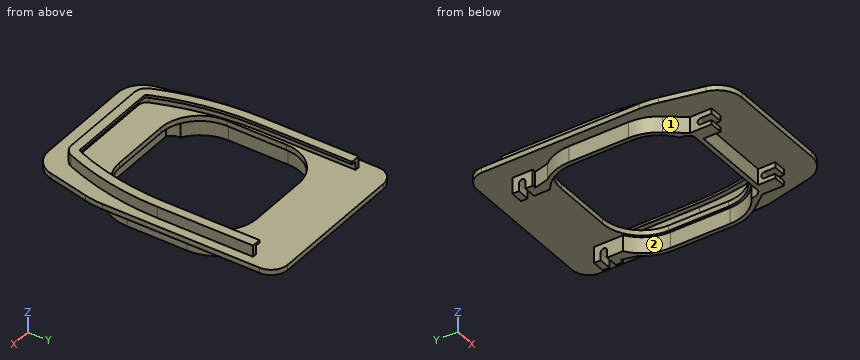
Autodesk Inventor part; units mm, degrees
ref_plane "YZ Plane" through (0, 0, 0) normal (1, 0, 0) x (0, 1, 0)
ref_plane "XZ Plane" through (0, 0, 0) normal (0, 1, 0) x (-1, 0, 0)
ref_plane "XY Plane" through (0, 0, 0) normal (0, 0, 1) x (1, 0, 0)
sketch "Skizze1" plane through (0, 0, 0) normal (0, 0, 1) x (1, 0, 0)
  line L0 (-33.4, 0) -> (33.4, 0)
  line L1 (41.4, -8) -> (41.4, -84.0456)
  line L2 (40.4201, -92.8453) -> (35.956, -112.6399)
  line L3 (24.25, -122) -> (-24.25, -122)
  line L4 (-35.956, -112.6399) -> (-40.4201, -92.8453)
  line L5 (-41.4, -84.0456) -> (-41.4, -8)
  line L6 (0, 0) -> (0, -122) construction
  arc A0 (-41.4, -84.0456) -> (-40.4201, -92.8453) centre (-1.4, -84.0456) ccw
  arc A1 (40.4201, -92.8453) -> (41.4, -84.0456) centre (1.4, -84.0456) ccw
  arc A2 (-35.956, -112.6399) -> (-24.25, -122) centre (-24.25, -110) ccw
  arc A3 (24.25, -122) -> (35.956, -112.6399) centre (24.25, -110) ccw
  arc A4 (-33.4, 0) -> (-41.4, -8) centre (-33.4, -8) ccw
  arc A5 (41.4, -8) -> (33.4, 0) centre (33.4, -8) ccw
  point P0 (33.8452, -122)
  point P1 (-33.8452, -122)
  point P2 (-41.4, -88.5)
  dimension "d1" = 82.8
  dimension "d2" = 122
  dimension "d3" = 33.5
  dimension "d4" = 40
  dimension "d5" = 12
  dimension "d6" = 8
  dimension "d15" = 48.5
extrude "Extrusion1" add sketch "Skizze1" along normal blind 2.6
sketch "Skizze2" plane through (0, 0, 2.6) normal (0, 0, 1) x (1, 0, 0)
  line L0 (-36.8, -14.4) -> (-36.8, -60.5202)
  arc A0 (-36.8, -60.5202) -> (-27.5742, -108.62) centre (93.2, -60.5202) ccw
  line L1 (-22, -112.4) -> (22, -112.4)
  line L2 (36.8, -14.4) -> (36.8, -60.5202)
  arc A1 (27.5742, -108.62) -> (36.8, -60.5202) centre (-93.2, -60.5202) ccw
  line L3 (-36.8, -60.5202) -> (36.8, -60.5202) construction
  line L4 (-36.8, -14.4) -> (36.8, -14.4) construction
  line L5 (0, 0) -> (0, -122) construction
  line L6 (-24.25, -122) -> (24.25, -122) construction
  arc A2 (-27.5742, -108.62) -> (-22, -112.4) centre (-22, -106.4) ccw
  arc A3 (22, -112.4) -> (27.5742, -108.62) centre (22, -106.4) ccw
  line L7 (41.4, -84.0456) -> (41.4, -8) construction
  line L8 (-41.4, -8) -> (-41.4, -84.0456) construction
  line L9 (-34.8, -60.5202) -> (-34.8, -14.4)
  line L10 (34.8, -14.4) -> (34.8, -60.5202)
  arc A4 (25.7161, -107.88) -> (34.8, -60.5202) centre (-93.2, -60.5202) ccw
  arc A5 (22, -110.4) -> (25.7161, -107.88) centre (22, -106.4) ccw
  line L11 (22, -110.4) -> (-22, -110.4)
  arc A6 (-25.7161, -107.88) -> (-22, -110.4) centre (-22, -106.4) ccw
  arc A7 (-34.8, -60.5202) -> (-25.7161, -107.88) centre (93.2, -60.5202) ccw
  line L12 (-36.8, -14.4) -> (-34.8, -14.4)
  line L13 (34.8, -14.4) -> (36.8, -14.4)
  point P0 (-25.9993, -112.4)
  point P1 (25.9993, -112.4)
  point P2 (0, -14.4)
  dimension "d9" = 6
  dimension "d10" = 6
  dimension "d11" = 130
  dimension "d12" = 4.6
  dimension "d13" = 9.6
  dimension "d14" = 44
  dimension "d16" = 14.4
  dimension "d17" = 2
extrude "Extrusion2" add sketch "Skizze2" along normal blind 5.5
sketch "Skizze3" plane through (-36.8, -14.4, 2.6) normal (0, 1, 0) x (1, 0, 0)
  line L0 (2, -4.2) -> (4.5, -4.2)
  line L1 (4.5, -4.2) -> (4.5, -5.5)
  line L2 (4.5, -5.5) -> (2, -5.5)
  line L3 (2, -5.5) -> (2, -4.2)
  line L4 (0, 0) -> (0, -5.5)
  point P0 (36.8, 2.6)
  dimension "d20" = 4.5
  dimension "d21" = 1.3
sketch "Skizze4" plane through (0, 0, 8.1) normal (0, 0, 1) x (1, 0, 0)
  line L0 (-34.8, -60.5202) -> (-34.8, -14.4)
  arc A0 (-34.8, -60.5202) -> (-25.7161, -107.88) centre (93.2, -60.5202) ccw
  arc A1 (-25.7161, -107.88) -> (-22, -110.4) centre (-22, -106.4) ccw
  line L1 (22, -110.4) -> (-22, -110.4)
  arc A2 (22, -110.4) -> (25.7161, -107.88) centre (22, -106.4) ccw
  arc A3 (25.7161, -107.88) -> (34.8, -60.5202) centre (-93.2, -60.5202) ccw
  line L2 (34.8, -14.4) -> (34.8, -60.5202)
  point P0 (0, 0)
sketch3d "3D-Skizze1"
  line L0 (-34.8, -14.4, 8.1) -> (-34.8, -60.5202, 8.1)
  arc A0 (-34.8, -60.5202, 8.1) -> (-25.7161, -107.88, 8.1) centre (93.2, -60.5202, 8.1) ccw
  arc A1 (-25.7161, -107.88, 8.1) -> (-22, -110.4, 8.1) centre (-22, -106.4, 8.1) ccw
  line L1 (-22, -110.4, 8.1) -> (22, -110.4, 8.1)
  arc A2 (22, -110.4, 8.1) -> (25.7161, -107.88, 8.1) centre (22, -106.4, 8.1) ccw
  arc A3 (25.7161, -107.88, 8.1) -> (34.8, -60.5202, 8.1) centre (-93.2, -60.5202, 8.1) ccw
  line L2 (34.8, -60.5202, 8.1) -> (34.8, -14.4, 8.1)
sweep "Sweeping1" add profiles "Skizze3" path "3D-Skizze1"
sketch "Skizze5" plane through (0, 0, 0) normal (0, 0, -1) x (-1, 0, 0)
  line L0 (-36.4, -24.7) -> (36.4, -24.7)
  line L1 (36.4, -24.7) -> (36.4, -97.5)
  line L2 (36.4, -97.5) -> (-36.4, -97.5)
  line L3 (-36.4, -97.5) -> (-36.4, -24.7)
  line L4 (-36.4, -24.7) -> (36.4, -97.5) construction
  line L5 (36.4, -24.7) -> (-36.4, -97.5) construction
  circle A0 centre (14.4, -46.7) radius 22 construction
  line L6 (0, 0) -> (0, -122) construction
  line L7 (24.25, -122) -> (-24.25, -122) construction
  line L8 (34.4, -26.7) -> (-34.4, -26.7)
  line L9 (-34.4, -26.7) -> (-34.4, -95.5)
  line L10 (-34.4, -95.5) -> (34.4, -95.5)
  line L11 (34.4, -95.5) -> (34.4, -26.7)
  line L12 (34.4, -26.7) -> (-34.4, -95.5) construction
  line L13 (-34.4, -26.7) -> (34.4, -95.5) construction
  circle A1 centre (-14.4, -46.7) radius 22 construction
  circle A2 centre (-14.4, -75.5) radius 22 construction
  circle A3 centre (14.4, -75.5) radius 22 construction
  line L14 (41.4, -8) -> (41.4, -84.0456) construction
  arc A4 (-36.4, -75.5) -> (-14.4, -97.5) centre (-14.4, -75.5) ccw
  arc A5 (-14.4, -24.7) -> (-36.4, -46.7) centre (-14.4, -46.7) ccw
  arc A6 (36.4, -46.7) -> (14.4, -24.7) centre (14.4, -46.7) ccw
  arc A7 (14.4, -97.5) -> (36.4, -75.5) centre (14.4, -75.5) ccw
  line L15 (-25.3, -97.5) -> (-19.1, -97.5)
  line L16 (-19.1, -97.5) -> (-19.1, -108)
  line L17 (-19.1, -108) -> (-25.3, -108)
  line L18 (-25.3, -108) -> (-25.3, -97.5)
  line L19 (19.1, -97.5) -> (25.3, -97.5)
  line L20 (25.3, -97.5) -> (25.3, -108)
  line L21 (25.3, -108) -> (19.1, -108)
  line L22 (19.1, -108) -> (19.1, -97.5)
  line L23 (-19.1, -108) -> (19.1, -108) construction
  arc A8 (-14.4, -26.7) -> (-34.4, -46.7) centre (-14.4, -46.7) ccw
  arc A9 (34.4, -46.7) -> (14.4, -26.7) centre (14.4, -46.7) ccw
  arc A10 (14.4, -95.5) -> (34.4, -75.5) centre (14.4, -75.5) ccw
  arc A11 (-34.4, -75.5) -> (-14.4, -95.5) centre (-14.4, -75.5) ccw
  line L24 (-25.3, -97.5) -> (-31.9034, -88.8279)
  line L25 (25.3, -97.5) -> (31.9034, -88.8279)
  line L26 (-19.1, -98.5) -> (19.1, -98.5)
  line L27 (19.1, -98.5) -> (19.1, -99.7)
  line L28 (19.1, -99.7) -> (-19.1, -99.7)
  line L29 (-19.1, -99.7) -> (-19.1, -98.5)
  arc A12 (-25.0991, -92.3976) -> (-19.1, -98.5) centre (-19.1, -92.5) ccw
  arc A13 (19.1, -98.5) -> (25.0991, -92.3976) centre (19.1, -92.5) ccw
  line L30 (-31.55, -16) -> (-25.45, -16)
  line L31 (-25.45, -16) -> (-25.45, -25.8)
  line L32 (-25.45, -25.8) -> (-31.55, -25.8)
  line L33 (-31.55, -25.8) -> (-31.55, -16)
  line L34 (25.45, -16) -> (31.55, -16)
  line L35 (31.55, -16) -> (31.55, -25.8)
  line L36 (31.55, -25.8) -> (25.45, -25.8)
  line L37 (25.45, -25.8) -> (25.45, -16)
  line L38 (-25.45, -16) -> (25.45, -16) construction
  line L39 (-29.75, -25.8) -> (-31.5142, -32.876)
  line L40 (29.75, -25.8) -> (31.5142, -32.876)
  line L41 (-29.75, -25.8) -> (-29.75, -30.94) construction
  line L42 (29.75, -25.8) -> (29.75, -30.94) construction
  line L43 (-25.45, -25.8) -> (-25.45, -30.0297)
  line L44 (25.45, -25.8) -> (25.45, -30.0297)
  line L45 (-33.25, -27.85) -> (33.25, -27.85)
  line L46 (33.25, -27.85) -> (33.25, -94.35)
  line L47 (33.25, -94.35) -> (-33.25, -94.35)
  line L48 (-33.25, -94.35) -> (-33.25, -27.85)
  line L49 (-33.25, -27.85) -> (33.25, -94.35) construction
  line L50 (33.25, -27.85) -> (-33.25, -94.35) construction
  circle A14 centre (-14.4, -75.5) radius 18.85
  circle A15 centre (-14.4, -46.7) radius 18.85
  circle A16 centre (14.4, -46.7) radius 18.85
  circle A17 centre (14.4, -75.5) radius 18.85
  point P0 (0, -61.1)
  point P1 (0, -24.7)
  point P2 (0, -108)
  point P3 (0, -16)
  point P4 (34.4, -46.7)
  point P5 (34.4, -75.5)
  point P6 (22.4166, -97.5)
  point P7 (-22.4166, -97.5)
  point P8 (-34.4, -75.5)
  point P9 (-34.4, -46.7)
  point P10 (-33.25, -40.0159)
  point P11 (-33.25, -82.1841)
  point P12 (-21.0841, -94.35)
  point P13 (21.0841, -94.35)
  point P14 (33.25, -82.1841)
  point P15 (33.25, -40.0159)
  point P16 (21.0841, -27.85)
  point P17 (-21.0841, -27.85)
  point P18 (14.4, -27.85)
  point P19 (-14.4, -27.85)
  point P20 (-33.25, -46.7)
  point P21 (-33.25, -75.5)
  point P22 (-14.4, -94.35)
  point P23 (14.4, -94.35)
  point P24 (33.25, -75.5)
  point P25 (33.25, -46.7)
  dimension "d25" = 2
  dimension "d26" = 22
  dimension "d27" = 5
  dimension "d29" = 6.2
  dimension "d30" = 6.2
  dimension "d31" = 38.2
  dimension "d33" = 1.2
  dimension "d34" = 3
  dimension "d35" = 6
  dimension "d36" = 6
  dimension "d37" = 63.1
  dimension "d38" = 6.1
  dimension "d39" = 6.1
  dimension "d40" = 92
  dimension "d41" = 9.8
  dimension "d42" = 37.287
  dimension "d44" = 1.8
  dimension "d45" = 1.8
  dimension "d46" = 14
  dimension "d79" = 66.5
  dimension "d80" = 66.5
  dimension "d83" = 22.3
  dimension "d84" = 14
extrude "Extrusion3" add sketch "Skizze5" along normal blind 7.8 contours L31 L32 L33 L0 | L0 L33 L30 L31 | L37 L34 L35 L0 | L0 L35 L36 L37 | L43 L8 L39 L32 | L43 A5 L45 L39 L8 | L43 L45 A5 | L36 L40 L8 L44 | L8 L40 L45 A6 L44 | A6 L45 L44 | L45 L43 A8 L48 A5 | A5 L39 L45 | L45 L40 A6 | A6 L46 A9 L44 L45 | A5 L9 A4 L3 | L1 A7 L11 A6 | A5 L48 A8 L9 | L11 A9 L46 A6 | L9 A11 L48 A4 | A7 L46 A10 L11 | L24 L10 A12 L2 | L2 A12 L16 L17 L18 | L48 A11 A12 L47 A4 | L20 L21 L22 A13 L2 | L2 A13 L10 L25 | A7 L47 A13 A10 L46 | L2 L16 A12 | L24 L47 A4 A12 L10 | A4 L47 L24 | A13 L22 L2 | L10 A13 A7 L47 L25 | L25 L47 A7 | L2 L22 L26 L16 | L26 L22 L28 L16 | L47 A12 A4 | A7 A13 L47
sketch "Skizze6" plane through (31.55, -25.8, 0) normal (1, 0, 0) x (0, 0, -1)
  line L0 (0, 0) -> (7.8, 0) construction
  circle A0 centre (4.15, 5.05) radius 1.55
  line L1 (7.8, 9.8) -> (7.8, 0)
  line L2 (4.15, 3.5) -> (7.8, 3.5)
  line L3 (4.15, 6.6) -> (7.8, 6.6)
  line L4 (2.6, 5.05) -> (2.6, 0) construction
  circle A1 centre (4.15, -76.95) radius 1.55
  line L5 (2.6, -76.95) -> (2.6, -82.2)
  line L6 (0, -82.2) -> (7.8, -82.2) construction
  line L7 (2.6, -82.2) -> (5.7, -82.2)
  line L8 (5.7, -82.2) -> (5.7, -76.95)
  line L9 (4.15, -75.4) -> (7.8, -75.4) construction
  line L10 (7.8, -71.7) -> (7.8, -82.2) construction
  line L11 (4.15, -82.2) -> (4.15, -76.95) construction
  line L12 (7.8, -20.9) -> (7.8, -49.7) construction
  line L13 (4.15, 5.05) -> (4.15, -76.95) construction
  point P0 (0, 25.8)
  dimension "d49" = 3.1
  dimension "d50" = 3.5
  dimension "d76" = 6.8
  dimension "d77" = 3.1
  dimension "d78" = 5.2
extrude "Extrusion4" cut sketch "Skizze6" against normal through all
ref_plane "Arbeitsebene1" through (0, -75.5, 0) normal (1, 0, 0) x (0, 0, -1)
extrude "Extrusion5" cut sketch "Skizze5" against normal up to surface (2.6 mm away) contours L45 A16 A15 | A15 A16 A14 | A16 A17 A15 | A15 A16 | A15 A14 L48 | L46 A17 A16 | A16 A17 A14 A15 | A14 A15 A17 | A14 A15 | A17 A14 A16 | A16 A17 | A14 A17 L47 | A14 A17
equation "\"d9\" = d10"
equation "\"d30\" = d29"
equation "\"d36\" = d35"
properties part number "daVinciTool_Aufnahme" material "PMMA-Kunststoff"
Check sheet for the modelled part. Datum: model origin and axes. Units: mm. Face numbers are marked on the shaded views. Round coordinates to 2 decimals unless told otherwise and drop trailing zeros. Loops run counter-clockwise (first coordinate to the right, second up) from the corner with the lowest first, then second, coordinate; pieces in that order, holes last. Notation, with made-up numbers: (77, 31.5) -> (119, 31.5) arc R11 cw to (119, 45.5) -> close; hole circle Ø6 at (14, 63.5). An arc over 180 degrees is marked (long way). Put each result on its own line as item: value. Start each with the question number.
1. Gauge pin test, flat ends, axial feed: pin 1 (4 mm diameter, centred on y = -64, z = -4, fed in from +X); pin 2 (2.5 mm diameter, centred on x = -20.5, y = -105, fed in from +Z); pin 3 (1 mm diameter, centred on x = 33.5, z = 7.5, fed in from +Y). Record the tip position at first contact, or that the pin passes through.
2. Draft check along X on the marked faces 1 and 2. Enter one of: +X half, -X half, draft (parallel to the pull), parting line (faces both ways), or undercut.
3. Section check B-B (z = 4.25). Enter the section's corners in (x, y), plus the area to 3 significant figures.
4. Scan lines: probe 1 along X at (y, z) = (-59, 1.25); probe 2 along X at (y, z) = (-18.5, -6.5); probe 3 along Z at (x, y) = (-10, -109). Record each from-to range of solid material in increasing order.
5. Section check A-A (x = 5). Enter the section's corners in (y, z), plus the area to 3 significant figures.
6. Section check C-C (y = -20.75). Enter the section's corners in (x, z).
7. Section check D-D (y = -70). Enter the section's corners in (x, z), plus the area to 3 significant figures.
Findings:
1. pin 1: stops at x = 36.4
1. pin 2: stops at z = 2.6
1. pin 3: stops at y = -14.4
2. face 1: -X half
2. face 2: undercut
3. outline: (-36.8, -60.52) arc R130 ccw to (-27.57, -108.62) arc R6 ccw to (-22, -112.4) -> (22, -112.4) arc R6 ccw to (27.57, -108.62) arc R130 ccw to (36.8, -60.52) -> (36.8, -14.4) -> (34.8, -14.4) -> (34.8, -60.52) arc R128 cw to (25.72, -107.88) arc R4 cw to (22, -110.4) -> (-22, -110.4) arc R4 cw to (-25.72, -107.88) arc R128 cw to (-34.8, -60.52) -> (-34.8, -14.4) -> (-36.8, -14.4) -> close
3. area: 492 mm^2
4. probe 1: x = -41.4 to -33.25, 33.25 to 41.4
4. probe 2: x = -31.55 to -25.45, 25.45 to 31.55
4. probe 3: z = 0 to 2.6, 6.8 to 8.1
5. outline: (-122, 0) -> (-99.7, 0) -> (-99.7, -7.8) -> (-97.5, -7.8) -> (-97.5, 0) -> (-94.35, 0) -> (-94.35, 2.6) -> (-110.4, 2.6) -> (-110.4, 6.8) -> (-107.9, 6.8) -> (-107.9, 8.1) -> (-112.4, 8.1) -> (-112.4, 2.6) -> (-122, 2.6) -> close; (-27.85, 0) -> (0, 0) -> (0, 2.6) -> (-27.85, 2.6) -> close
5. area: 176 mm^2
6. outline: (-41.4, 0) -> (-31.55, 0) -> (-31.55, -2.6) -> (-25.45, -2.6) -> (-25.45, 0) -> (25.45, 0) -> (25.45, -2.6) -> (31.55, -2.6) -> (31.55, 0) -> (41.4, 0) -> (41.4, 2.6) -> (36.8, 2.6) -> (36.8, 8.1) -> (32.3, 8.1) -> (32.3, 6.8) -> (34.8, 6.8) -> (34.8, 2.6) -> (-34.8, 2.6) -> (-34.8, 6.8) -> (-32.3, 6.8) -> (-32.3, 8.1) -> (-36.8, 8.1) -> (-36.8, 2.6) -> (-41.4, 2.6) -> close
7. outline: (-41.4, 0) -> (-36.4, 0) -> (-36.4, -7.8) -> (-34.4, -7.8) -> (-34.4, 0) -> (-33.25, 0) -> (-33.25, 2.6) -> (-34.45, 2.6) -> (-34.45, 6.8) -> (-31.94, 6.8) -> (-31.94, 8.1) -> (-36.45, 8.1) -> (-36.45, 2.6) -> (-41.4, 2.6) -> close; (31.94, 6.8) -> (34.45, 6.8) -> (34.45, 2.6) -> (33.25, 2.6) -> (33.25, 0) -> (34.4, 0) -> (34.4, -7.8) -> (36.4, -7.8) -> (36.4, 0) -> (41.4, 0) -> (41.4, 2.6) -> (36.45, 2.6) -> (36.45, 8.1) -> (31.94, 8.1) -> close
7. area: 102 mm^2
